from build123d import *

# Parameters (mm, degrees)
F0_W          = 129.1844
F0_H          = 128.892914
F0_W_2        = 99.1844
F0_H_2        = 98.892914
F1_DEPTH      = 3
F2_W          = 135.1844
F2_H          = 134.892914
F2_W_2        = 129.1844
F2_H_2        = 128.892914
F3_DEPTH      = 25.4
F3_DEPTH_BACK = 25.4


with BuildPart() as f1:
    # F0 (on Top) → F1 (new body)
    with BuildSketch(Plane.XY):
        Rectangle(F0_W, F0_H)
        Rectangle(F0_W_2, F0_H_2, mode=Mode.SUBTRACT)
    extrude(amount=F1_DEPTH)

    # F2 (on Top) → F3 (join, two sides)
    with BuildSketch(Plane.XY) as f3_sk:
        Rectangle(F2_W, F2_H)
        Rectangle(F2_W_2, F2_H_2, mode=Mode.SUBTRACT)
    extrude(amount=F3_DEPTH)
    extrude(f3_sk.sketch, amount=-F3_DEPTH_BACK)


solid = f1.part
Work out the finished part from the listing and answer in its coordinate system (mm). A direction names the side the tool comes from. Round coordinates to 2 decimals unless told otherwise and drop trailing zeros. Write each loop counter-clockwise with the first axis right and the second up, starting at its lowest first coordinate (ties: lowest second). Pieces come first, ordered by that corner, then holes. Notation, with made-up numbers: (-37, 7) -> (-3, 7) arc R18 ccw to (-3, 18) -> close; hole circle Ø10 at (-19, -33.5). An arc over 180 degrees is marked (long way). Write each question's results on one line, items separated by ' | '.
Item 1: A flat-ended cylindrical pin translates along its axis: P1, Ø12, axis at x = 52, y = 14.5, coming from the -Z side. Find the tip coordinate at first contact, or state that the pin passes through.
Result set:
P1: z = 0
Item 2: Find the intervals of material crossed by line 1 along X through (y, z) = (-48, -9); line 2 along Y through (x, z) = (-2.5, 3.5); line 3 along Y through (x, z) = (22, 2), in increasing order. Write a range as [from, to].
Result set:
line 1: [-67.59, -64.59], [64.59, 67.59] | line 2: [-67.45, -64.45], [64.45, 67.45] | line 3: [-67.45, -49.45], [49.45, 67.45]
Item 3: A cutting plane is placed at A-A, the plane y = -24.5. Determine the outline of the cut face in (x, z).
Result set:
outline: (-67.59, -25.4) -> (-64.59, -25.4) -> (-64.59, 0) -> (-49.59, 0) -> (-49.59, 3) -> (-64.59, 3) -> (-64.59, 25.4) -> (-67.59, 25.4) -> close; (49.59, 0) -> (64.59, 0) -> (64.59, -25.4) -> (67.59, -25.4) -> (67.59, 25.4) -> (64.59, 25.4) -> (64.59, 3) -> (49.59, 3) -> close
Item 4: A cutting plane is placed at C-C, the plane z = -7. Determine the outline of the cut face in (x, y).
Result set:
outline: (-67.59, -67.45) -> (67.59, -67.45) -> (67.59, 67.45) -> (-67.59, 67.45) -> close; hole (-64.59, -64.45) -> (64.59, -64.45) -> (64.59, 64.45) -> (-64.59, 64.45) -> close
Item 5: Which of the six approach directions +Z, -Z, +X, -X, +Y, -Y give full straight-line access (tool end or side, diameter ignored) to faces 4 (the face through (-1, -64.446, 14)), 5 (the face through (-1, 49.446, 1)), 6 (the face through (-1, 67.446, 0)), 7 (the face through (-1, -64.446, -13)), 8 (the face through (-5, -65, -25.4))?
Result set:
face 4: +Z | face 5: +Z, -Z | face 6: +Z, -Z, +X, -X, +Y | face 7: -Z | face 8: -Z, +X, -X, +Y, -Y
Item 6: A cutting plane is placed at B-B, the plane x = -30.5. Determine the outline of the cut face in (y, z), plus the area to 3 significant figures.
Result set:
outline: (-67.45, -25.4) -> (-64.45, -25.4) -> (-64.45, 0) -> (-49.45, 0) -> (-49.45, 3) -> (-64.45, 3) -> (-64.45, 25.4) -> (-67.45, 25.4) -> close; (49.45, 0) -> (64.45, 0) -> (64.45, -25.4) -> (67.45, -25.4) -> (67.45, 25.4) -> (64.45, 25.4) -> (64.45, 3) -> (49.45, 3) -> close | area: 395 mm^2
Item 7: The mould has two halves that part along X. Classify faces 1 (the face through (-5, -65, 25.4)), 2 (the face through (49.592, -1, 1)), 3 (the face through (67.592, -1, 0)): +X half, -X half, draft (parallel to the pull), parting line (faces both ways), or undercut.
Result set:
face 1: draft | face 2: undercut | face 3: +X half
Item 8: A cutting plane is placed at D-D, the plane x = 59. Determine the outline of the cut face in (y, z), plus the area to 3 significant figures.
Result set:
outline: (-67.45, -25.4) -> (-64.45, -25.4) -> (-64.45, 0) -> (64.45, 0) -> (64.45, -25.4) -> (67.45, -25.4) -> (67.45, 25.4) -> (64.45, 25.4) -> (64.45, 3) -> (-64.45, 3) -> (-64.45, 25.4) -> (-67.45, 25.4) -> close | area: 691 mm^2
